Check sheet for the modelled part. Datum: model origin and axes. Units: mm. A direction names the side the tool comes from. Round coordinates to 2 decimals unless told otherwise and drop trailing zeros. Loops run counter-clockwise (first coordinate to the right, second up) from the corner with the lowest first, then second, coordinate; pieces in that order, holes last. Notation, with made-up numbers: (28, 33) - (39, 33) arc R21 cw to (39, 63) - close; hole circle Ø11 at (6.25, -18.5). An arc over 180 degrees is marked (long way). Return JSON: item names as keys, results as strings.
Autodesk Inventor part; units mm, degrees
ref_plane "YZ Plane" through (0, 0, 0) normal (1, 0, 0) x (0, 1, 0)
ref_plane "XZ Plane" through (0, 0, 0) normal (0, 1, 0) x (-1, 0, 0)
ref_plane "XY Plane" through (0, 0, 0) normal (0, 0, 1) x (1, 0, 0)
sketch "Sketch1" plane through (0, 0, 0) normal (0, 0, 1) x (1, 0, 0)
  line L0 (0, 0) -> (-13.377, 0)
  line L1 (0, 0) -> (0, 26.67)
  line L2 (0, 26.67) -> (26.67, 0)
  line L3 (26.67, 0) -> (0, 0)
  dimension "d0" = 26.67
extrude "Extrusion1" add sketch "Sketch1" along normal mid plane 7.366
sketch "Sketch3" plane through (0, 0, 0) normal (0, 0, 1) x (1, 0, 0)
  line L0 (0, 26.67) -> (26.67, 0)
  line L1 (0, 0) -> (0, 26.67)
  line L2 (26.67, 0) -> (0, 0)
  line L3 (1.524, 25.146) -> (1.524, 1.524)
  line L4 (1.524, 1.524) -> (25.146, 1.524)
  line L5 (1.524, 25.146) -> (25.146, 1.524)
  dimension "d3" = 1.524
  dimension "d4" = 1.524
extrude "Extrusion2" cut sketch "Sketch3" against normal mid plane 4.318 contours L0 L4 L3
fillet "Fillet1" radius 1.524 3 edges at (0, 26.67, 0) (0, 0, 0) (26.67, 0, 0)
fillet "Fillet2" radius 1.016 6 edges at (0.4464, 0.4464, 3.683) (12.2574, 0, 3.683) (24.3987, 0.9408, 3.683) (13.335, 13.335, 3.683) (0.9408, 24.3987, 3.683) (0, 12.2574, 3.683)
fillet "Fillet3" radius 1.016 6 edges at (0.9408, 24.3987, -3.683) (13.335, 13.335, -3.683) (24.3987, 0.9408, -3.683) (12.2574, 0, -3.683) (0.4464, 0.4464, -3.683) (0, 12.2574, -3.683)
equation "\"d0\" = edgeSize"
equation "\"d1\" = partThickness"
equation "\"d3\" = edgeThickness"
equation "\"d4\" = edgeThickness"
equation "\"d5\" = mirrorThickness"
equation "\"d7\" = filetForCorners"
equation "\"d8\" = filetForFlat"
equation "\"d9\" = filetForFlat"
equation "\"edgeSize\" = 26.67"
equation "\"wallThickness\" = 1.524"
equation "\"mirrorThickness\" = 4.318"
equation "\"partThickness\" = mirrorThickness + 2 * wallThickness"
equation "\"edgeThickness\" = 1.524"
equation "\"filetForCorners\" = 1.524"
equation "\"filetForFlat\" = 1.016"
properties part number "Mirror Corner"
Q1. Draft check along Z on faces 1 (the face through (12, 0, 0)), 2 (the face through (1.524, 13, 0)), 3 (the face through (13, 1.524, 0)), 4 (the face through (12.41, 0.29, -3.38)). Enter one of: released by +Z, released by -Z, zero draft, split by the parting line, or undercut.
Answer key:
{"face 1": "zero draft", "face 2": "undercut", "face 3": "undercut", "face 4": "released by -Z"}
Q2. Tool access check on faces 5 (the face through (12.11, 0.29, 3.38)), 6 (the face through (10, 11, 2.159)). Record the directions out of +Z, -Z, +X, -X, +Y, -Y that give a thin tool (end or side, any length) a straight path to the whole face; none if there is none.
Answer key:
{"face 5": "+Z, +X, -X, -Y", "face 6": "+X, +Y"}
Q3. Sectioned sample at A-A (z = 1.75). Enter the section's corners in (x, y).
Answer key:
{"outline": "(0, 1.52) arc R1.52 ccw to (1.52, 0) - (22.99, 0) arc R1.52 ccw to (24.51, 1.52) - (1.52, 1.52) - (1.52, 24.51) arc R1.52 ccw to (0, 22.99) - close"}
Q4. Scan lines: probe 1 along Z at (x, y) = (5.75, 5); probe 2 along Y at (x, z) = (18.5, 1.5). Record each from-to range of solid material in increasing order. Write a range as [from, to].
Answer key:
{"probe 1": "z = [-3.68, -2.16], [2.16, 3.68]", "probe 2": "y = [0, 1.52]"}
